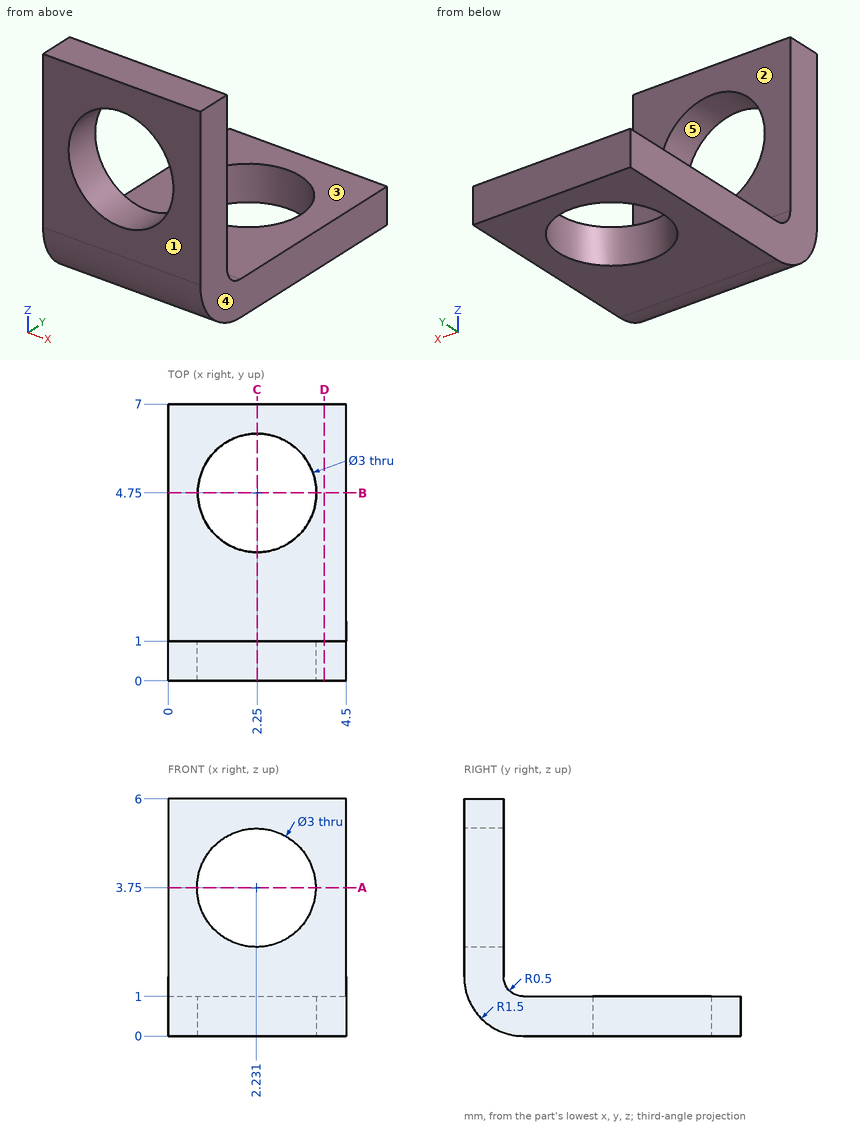
Study the drawing (mm; zero at the part's minimum x, y, z) and answer. A direction names the side the tool comes from. Coordinates: 2 decimals unless noted, no trailing zeros. Loops run counter-clockwise (first coordinate to the right, second up) from the corner with the lowest first, then second, coordinate; pieces in that order, holes last. Notation, with made-up numbers: M -0.75,24 L 39.25,24 A28 ccw 39.25,44 Z; hole C 66.5,14 d8. An arc over 180 degrees is marked long. Answer as a JSON object with one key per item and string values. Group by question number.
Item 1: Section A-A (z = 3.75) is taken. Write down the section's boundary in (x, y), and give its area (3 significant figures).
Item 2: Section D-D (x = 3.95) is taken. Write down the section's boundary in (y, z).
Item 3: Determine the mould class of the marked faces 3, 4 and 5 for opening direction X: +X half, -X half, draft (parallel to the pull), parting line (faces both ways), or undercut.
Item 4: Section C-C (x = 2.25) is taken. Write down the section's boundary in (y, z), and give its area (3 significant figures).
Item 5: Section B-B (y = 4.75) is taken. Write down the section's boundary in (x, z).
Item 6: This flat-tipped pin is pushed along its axis until it touches: P1, Ø1, axis at x = 4, y = 4.5, coming from the +Z side. Where does it stop, or does it pass through?
Item 7: Which of the six approach directions +Z, -Z, +X, -X, +Y, -Y give full straight-line access (tool end or side, diameter ignored) to the marked faces 1 and 2?
Item 8: Consider L1, parallel to X at y = 4.75, z = 0.8; L2, parallel to Z at x = 0.75, y = 2.75; L3, parallel to Z at x = 1.8, y = 0.5. Determine where each line is inside the solid, lowest interval first.
Solved:
{
 "1": {"outline": "M 0,0 L 0.73,0 L 0.73,1 L 0,1 Z; M 3.73,0 L 4.5,0 L 4.5,1 L 3.73,1 Z", "area": "1.50 mm2"},
 "2": {"outline": "M 0,1.5 A1.5 ccw 1.5,0 L 7,0 L 7,1 L 1.5,1 A0.5 cw 1,1.5 L 1,6 L 0,6 Z"},
 "3": {"face 3": "draft", "face 4": "+X half", "face 5": "undercut"},
 "4": {"outline": "M 0,1.5 A1.5 ccw 1.5,0 L 3.25,0 L 3.25,1 L 1.5,1 A0.5 cw 1,1.5 L 1,2.25 L 0,2.25 Z; M 0,5.25 L 1,5.25 L 1,6 L 0,6 Z; M 6.25,0 L 7,0 L 7,1 L 6.25,1 Z", "area": "5.57 mm2"},
 "5": {"outline": "M 0,0 L 0.75,0 L 0.75,1 L 0,1 Z; M 3.75,0 L 4.5,0 L 4.5,1 L 3.75,1 Z"},
 "6": {"P1": "stops at z = 1"},
 "7": {"face 1": "+Z, -Z, +X, -X, -Y", "face 2": "+Z, +X, -X, +Y"},
 "8": {"L1": "x = 0 to 0.75, 3.75 to 4.5", "L2": "z = 0 to 1", "L3": "z = 0.38 to 2.31, 5.19 to 6"}
}
